from build123d import *

# Parameters (mm, degrees)
SKETCH1_R           = 1
BOSS_EXTRUDE1_DEPTH = 1.2
SKETCH2_W           = 27.7
SKETCH2_H           = 29.450740724
BOSS_EXTRUDE2_DEPTH = 2


with BuildPart() as part:
    # Sketch1 → Boss-Extrude1 (new body)
    with BuildSketch(Plane(origin=(0, 0, 0), x_dir=(1, 0, 0), z_dir=(0, 1, 0))):
        with BuildLine():
            ThreePointArc((0, 37.72), (0.439339828, 38.780660172), (1.5, 39.22))
            Line((1.5, 39.22), (26.2, 39.22))
            ThreePointArc((26.2, 39.22), (27.260660172, 38.780660172), (27.7, 37.72))
            Line((27.7, 37.72), (27.7, 1.5))
            ThreePointArc((27.7, 1.5), (27.260660172, 0.439339828), (26.2, 0))
            Line((26.2, 0), (1.5, 0))
            ThreePointArc((1.5, 0), (0.439339828, 0.439339828), (0, 1.5))
            Line((0, 1.5), (0, 37.72))
        make_face()
        with Locations(Location((25.2, 2.5, 0), (0, 0, 270))):
            Circle(SKETCH1_R, mode=Mode.SUBTRACT)
        with Locations(Location((3.286079962, 2.5, 0), (0, 0, 270))):
            Circle(SKETCH1_R, mode=Mode.SUBTRACT)
        with Locations(Location((25.51, 37.72, 0), (0, 0, 270))):
            Circle(SKETCH1_R, mode=Mode.SUBTRACT)
        with Locations(Location((2.19, 37.72, 0), (0, 0, 270))):
            Circle(SKETCH1_R, mode=Mode.SUBTRACT)
    extrude(amount=BOSS_EXTRUDE1_DEPTH)

    # Sketch2 → Boss-Extrude2 (add)
    with BuildSketch(Plane(origin=(0, 1.2, 0), x_dir=(1, 0, 0), z_dir=(0, 1, 0))):
        with Locations((13.85, 19.725370362)):
            Rectangle(SKETCH2_W, SKETCH2_H)
    extrude(amount=BOSS_EXTRUDE2_DEPTH)


solid = part.part
Verification items for the finished model (mm, model axes). A direction names the side the tool comes from. Give positions to 0.01 mm unless a question says otherwise; leave off trailing zeros. Loops run counter-clockwise (first coordinate to the right, second up) from the corner with the lowest first, then second, coordinate; pieces in that order, holes last. Notation, with made-up numbers: (31, -11.75) - (83, -11.75) arc R23 cw to (83, 6.25) - close; hole circle Ø9 at (71, 27). An arc over 180 degrees is marked (long way). Write item = value, one per line. Start each with the question number.
Q1. Thickness scan on line 1 (X direction, y = 0.5, z = -2.5); line 2 (X direction, y = 0.9, z = -37.72); line 3 (Y direction, x = 19, z = -37). Record the ranges inside material, lowest first.
Q2. Depth check by flat-ended pin: P1, Ø2.5, axis at x = 3.29, z = -2.5, coming from the +Y side; P2, Ø0.6, axis at x = 11.5, y = 2, coming from the +Z side; P3, Ø0.6, axis at x = 16.5, y = 2.5, coming from the -Z side. Enter the tip coordinate at first touch or a pass-through.
Q3. Tool access check on faces 4 (the face through (14, 3.2, -20)), 5 (the face through (14, 1.2, -37)), 6 (the face through (14, 1.2, -3)). Record the directions out of +Z, -Z, +X, -X, +Y, -Y that give a thin tool (end or side, any length) a straight path to the whole face; none if there is none.
Q4. Mould release check, pull along Z, two halves, no side actions. Record for faces 1 (the face through (27.7, 2, -20)), 2 (the face through (1.214, 0.592, -37.937)), 3 (the face through (14, 2, -34.451)): released by +Z, released by -Z, zero draft, split by the parting line, or undercut.
Q5. Cross-section at A-A, the plane z = -2.5. Enter the section's corners in (x, y), and give its area (3 significant figures).
Q6. Cross-section at C-C, the plane y = 2.7. Enter the section's corners in (x, z).
Q7. Cross-section at D-D, the plane z = -35.5. Enter the section's corners in (x, y).
Q8. Cross-section at B-B, the plane x = 5.75. Enter the section's corners in (y, z), and give its area (3 significant figures).
Answer key:
q1.line_1 = 0 to 2.29, 4.29 to 24.2, 26.2 to 27.7
q1.line_2 = 0 to 1.19, 3.19 to 24.51, 26.51 to 27.7
q1.line_3 = 0 to 1.2
q2.P1 = 1.2
q2.P2 = -5
q2.P3 = -34.45
q3.face_4 = +Z, -Z, +X, -X, +Y
q3.face_5 = -Z, +X, -X, +Y
q3.face_6 = +Z, +X, -X, +Y
q4.face_1 = zero draft
q4.face_2 = undercut
q4.face_3 = released by -Z
q5.outline = (0, 0) - (2.29, 0) - (2.29, 1.2) - (0, 1.2) - close; (4.29, 0) - (24.2, 0) - (24.2, 1.2) - (4.29, 1.2) - close; (26.2, 0) - (27.7, 0) - (27.7, 1.2) - (26.2, 1.2) - close
q5.area = 28.4 mm^2
q6.outline = (0, -34.45) - (27.7, -34.45) - (27.7, -5) - (0, -5) - close
q7.outline = (0, 0) - (27.7, 0) - (27.7, 1.2) - (0, 1.2) - close
q8.outline = (0, -39.22) - (1.2, -39.22) - (1.2, -34.45) - (3.2, -34.45) - (3.2, -5) - (1.2, -5) - (1.2, 0) - (0, 0) - close
q8.area = 106 mm^2
